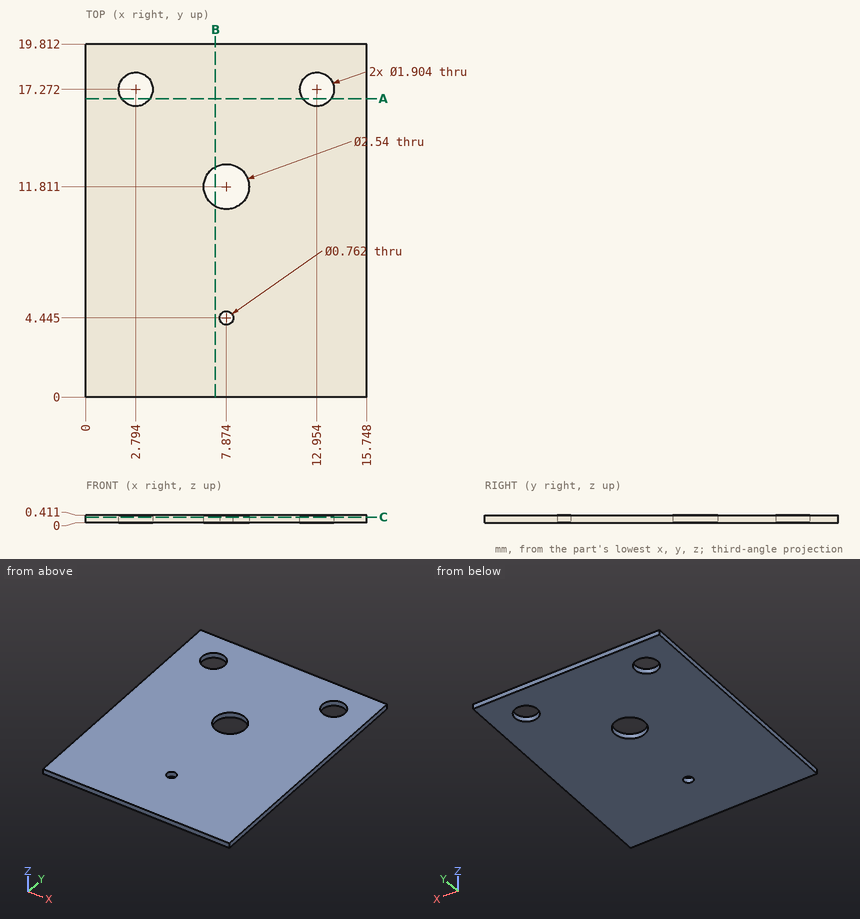
Here's the drawing with two shaded views (mm, measured from the low corner). I have some questions. Coordinates: 2 decimals unless noted, no trailing zeros. Write each loop counter-clockwise with the first axis right and the second up, starting at its lowest first coordinate (ties: lowest second). Pieces come first, ordered by that corner, then holes. Notation, with made-up numbers: M -22,55 L -3,55 A15 ccw -3,80 Z; hole C 17,53 d2. An arc over 180 degrees is marked long. Answer as CSV lines item,"result". Start each with the question number.
1) I want a section at C-C, the plane z = 0.3. Please give me the cut outline in (x, y) (1 decimal).
2) I want a section at B-B, the plane x = 7.25. Please give me the cut outline in (y, z) (1 decimal).
3) Please list where these lines run through material, in increasing order: line 1 (Y direction, x = 13, z = 0.35); line 2 (X direction, y = 17.5, z = 0.15); line 3 (Y direction, x = 13.25, z = 0.3). Write a range as from..to.
4) I want a section at A-A, the plane y = 16.75. Please give me the cut outline in (x, z).
Data:
1,outline,"M 0,0 L 15.7,0 L 15.7,19.8 L 0,19.8 Z; hole C 2.8,17.3 d1.9; hole C 7.9,11.8 d2.5; hole C 7.9,4.4 d0.8; hole C 13,17.3 d1.9"
2,outline,"M 0,0 L 10.7,0 L 10.7,0.4 L 0,0.4 Z; M 12.9,0 L 19.8,0 L 19.8,0.4 L 12.9,0.4 Z"
3,line 1,"y = 0..16.32, 18.22..19.81"
3,line 2,"x = 0..1.87, 3.72..12.03, 13.88..15.75"
3,line 3,"y = 0..16.37, 18.18..19.81"
4,outline,"M 0,0 L 2,0 L 2,0.41 L 0,0.41 Z; M 3.59,0 L 12.16,0 L 12.16,0.41 L 3.59,0.41 Z; M 13.75,0 L 15.75,0 L 15.75,0.41 L 13.75,0.41 Z"
